```python
from build123d import *

# Parameters (mm, degrees)
F0_R          = 3
F0_R_2        = 2.5
F1_DEPTH      = 246.7
F2_R          = 2
F3_R          = 7
F6_DEPTH      = 30
F6_DEPTH_BACK = 30


# Not quite as in the source:
# - a feature names something its author has since deleted; it is built from what else it names


with BuildPart() as f1:
    # F0 (on Top) → F1 (new body)
    with BuildSketch(Plane.XY):
        with BuildLine():
            Line((18.15, -30), (30, -30))
            Line((30, -30), (30, -18.15))
            Line((30, -18.15), (27.5, -18.15))
            Line((27.5, -18.15), (27.5, -20.15))
            Line((27.5, -20.15), (21.5477069044, -20.15))
            ThreePointArc((21.5477069044, -20.15), (19.5, -15), (21.5477069044, -9.85))
            Line((21.5477069044, -9.85), (27.5, -9.85))
            Line((27.5, -9.85), (27.5, -11.85))
            Line((27.5, -11.85), (30, -11.85))
            Line((30, -11.85), (30, 11.85))
            Line((30, 11.85), (27.5, 11.85))
            Line((27.5, 11.85), (27.5, 9.85))
            Line((27.5, 9.85), (21.5477069044, 9.85))
            ThreePointArc((21.5477069044, 9.85), (19.5, 15), (21.5477069044, 20.15))
            Line((21.5477069044, 20.15), (27.5, 20.15))
            Line((27.5, 20.15), (27.5, 18.15))
            Line((27.5, 18.15), (30, 18.15))
            Line((30, 18.15), (30, 30))
            Line((30, 30), (18.15, 30))
            Line((18.15, 30), (18.15, 27.5))
            Line((18.15, 27.5), (20.15, 27.5))
            Line((20.15, 27.5), (20.15, 21.5477069044))
            ThreePointArc((20.15, 21.5477069044), (15, 19.5), (9.85, 21.5477069044))
            Line((9.85, 21.5477069044), (9.85, 27.5))
            Line((9.85, 27.5), (11.85, 27.5))
            Line((11.85, 27.5), (11.85, 30))
            Line((11.85, 30), (-11.85, 30))
            Line((-11.85, 30), (-11.85, 27.5))
            Line((-11.85, 27.5), (-9.85, 27.5))
            Line((-9.85, 27.5), (-9.85, 21.5477069044))
            ThreePointArc((-9.85, 21.5477069044), (-15, 19.5), (-20.15, 21.5477069044))
            Line((-20.15, 21.5477069044), (-20.15, 27.5))
            Line((-20.15, 27.5), (-18.15, 27.5))
            Line((-18.15, 27.5), (-18.15, 30))
            Line((-18.15, 30), (-30, 30))
            Line((-30, 30), (-30, 18.15))
            Line((-30, 18.15), (-27.5, 18.15))
            Line((-27.5, 18.15), (-27.5, 20.15))
            Line((-27.5, 20.15), (-21.5477069044, 20.15))
            ThreePointArc((-21.5477069044, 20.15), (-19.5, 15), (-21.5477069044, 9.85))
            Line((-21.5477069044, 9.85), (-27.5, 9.85))
            Line((-27.5, 9.85), (-27.5, 11.85))
            Line((-27.5, 11.85), (-30, 11.85))
            Line((-30, 11.85), (-30, -11.85))
            Line((-30, -11.85), (-27.5, -11.85))
            Line((-27.5, -11.85), (-27.5, -9.85))
            Line((-27.5, -9.85), (-21.5477069044, -9.85))
            ThreePointArc((-21.5477069044, -9.85), (-19.5, -15), (-21.5477069044, -20.15))
            Line((-21.5477069044, -20.15), (-27.5, -20.15))
            Line((-27.5, -20.15), (-27.5, -18.15))
            Line((-27.5, -18.15), (-30, -18.15))
            Line((-30, -18.15), (-30, -30))
            Line((-30, -30), (-18.15, -30))
            Line((-18.15, -30), (-18.15, -27.5))
            Line((-18.15, -27.5), (-20.15, -27.5))
            Line((-20.15, -27.5), (-20.15, -21.5477069044))
            ThreePointArc((-20.15, -21.5477069044), (-15, -19.5), (-9.85, -21.5477069044))
            Line((-9.85, -21.5477069044), (-9.85, -27.5))
            Line((-9.85, -27.5), (-11.85, -27.5))
            Line((-11.85, -27.5), (-11.85, -30))
            Line((-11.85, -30), (11.85, -30))
            Line((11.85, -30), (11.85, -27.5))
            Line((11.85, -27.5), (9.85, -27.5))
            Line((9.85, -27.5), (9.85, -21.5477069044))
            ThreePointArc((9.85, -21.5477069044), (15, -19.5), (20.15, -21.5477069044))
            Line((20.15, -21.5477069044), (20.15, -27.5))
            Line((20.15, -27.5), (18.15, -27.5))
            Line((18.15, -27.5), (18.15, -30))
        make_face()
        with Locations((-25, -25)):
            Circle(F0_R, mode=Mode.SUBTRACT)
        with Locations((-15, -15)):
            Circle(F0_R_2, mode=Mode.SUBTRACT)
        with Locations((25, -25)):
            Circle(F0_R, mode=Mode.SUBTRACT)
        with Locations((15, -15)):
            Circle(F0_R_2, mode=Mode.SUBTRACT)
        with Locations((-25, 25)):
            Circle(F0_R, mode=Mode.SUBTRACT)
        with Locations((-15, 15)):
            Circle(F0_R_2, mode=Mode.SUBTRACT)
        Polygon((-7, 22), (-7, 27.5), (0, 27.5), (7, 27.5), (7, 22), (10, 16), (10, 10), (16, 10), (22, 7), (27.5, 7), (27.5, 0), (27.5, -7), (22, -7), (16, -10), (10, -10), (10, -16), (7, -22), (7, -27.5), (0, -27.5), (-7, -27.5), (-7, -22), (-10, -16), (-10, -10), (-16, -10), (-22, -7), (-27.5, -7), (-27.5, 0), (-27.5, 7), (-22, 7), (-16, 10), (-10, 10), (-10, 16), align=None, mode=Mode.SUBTRACT)
        with Locations((15, 15)):
            Circle(F0_R_2, mode=Mode.SUBTRACT)
        with Locations((25, 25)):
            Circle(F0_R, mode=Mode.SUBTRACT)
    extrude(amount=F1_DEPTH)

    # F2
    f2_edges = [f1.edges().sort_by_distance(p)[0] for p in [
        (-7, 27.5, 123.35),
        (7, 27.5, 123.35),
    ]]
    fillet(f2_edges, radius=F2_R)

    # F3
    f3_edges = [f1.edges().sort_by_distance(p)[0] for p in [
        (-10, 16, 123.35),
        (10, 16, 123.35),
    ]]
    fillet(f3_edges, radius=F3_R)

    # F5 (on Front) → F6 (cut, two sides)
    with BuildSketch(Plane.XZ) as f6_sk:
        Polygon((-21.4844248466, -51.4844248466), (30, 0), (-30.7442165391, 60.7442165391), (-82.2286413857, 9.2597916926), align=None)
        Polygon((69.921577374, 205.311127478), (91.4664718921, 257.3251040235), (-8.4551054819, 298.7139765456), (-30, 246.7), align=None)
    extrude(amount=F6_DEPTH, mode=Mode.SUBTRACT)
    extrude(f6_sk.sketch, amount=-F6_DEPTH_BACK, mode=Mode.SUBTRACT)


solid = f1.part
```
Check sheet for the modelled part. Datum: model origin and axes. Units: mm. Give positions to 0.01 mm unless a question says otherwise; leave off trailing zeros. Order: outer loops, then holes, each group sorted by start corner. A loop starts at its lowest first (then second) coordinate and runs counter-clockwise, first axis right, second up. Notation, with made-up numbers: (43, -40) -> (87, -40) arc R24 ccw to (87, -13) -> close; hole circle Ø4 at (78, 48). An arc over 180 degrees is marked (long way). Return JSON: item names as keys, results as strings.
1. Mould release check, pull along X, two halves, no side actions. Record for faces 1 (the flat face through (-30, -24, 152)), 2 (the flat face through (0, -30, 127)), 3 (the flat face through (-19, 8.5, 143.3)), 4 (the flat face through (30, 24, 109)): +X half, -X half, draft (parallel to the pull), parting line (faces both ways), or undercut.
From the geometry:
{"face 1": "-X half", "face 2": "draft", "face 3": "undercut", "face 4": "+X half"}
2. Material ranges on probe 1 along X at (y, z) = (-15, 199); probe 2 along Y at (x, z) = (-25, 200.5); probe 3 along X at (y, z) = (4, 209.5), recorded low to high. Write a range as [from, to].
From the geometry:
{"probe 1": "[-19.5, -17.5], [-12.5, -10], [10, 12.5], [17.5, 19.5]", "probe 2": "[-30, -28], [-22, -20.15], [-9.85, -7], [7, 9.85], [20.15, 22], [28, 30]", "probe 3": "[-30, -27.5], [27.5, 30]"}
3. Cross-section at C-C, the plane z = 91. Count the separate pieces of the cut face and the enclosed holes in it, plus the area to 3 significant figures.
From the geometry:
{"separate pieces": "1", "enclosed holes": "9", "area": "1,080 mm^2"}
4. Cross-section at B-B, the plane y = -25. Record the cut outline in (x, z).
From the geometry:
{"outline": "(-30, 60) -> (-28, 58) -> (-28, 245.87) -> (-30, 246.7) -> close; (-22, 52) -> (-20.15, 50.15) -> (-20.15, 242.62) -> (-22, 243.39) -> close; (-9.85, 39.85) -> (-7, 37) -> (-7, 237.17) -> (-9.85, 238.35) -> close; (7, 23) -> (9.85, 20.15) -> (9.85, 230.19) -> (7, 231.37) -> close; (20.15, 9.85) -> (22, 8) -> (22, 225.16) -> (20.15, 225.93) -> close; (28, 2) -> (30, 0) -> (30, 221.85) -> (28, 222.68) -> close"}
5. Go/stop test with flat-tipped pins: P1, Ø1.8, axis at y = -13.5, z = 140.5, coming from the +X side; P2, Ø10, axis at x = -10, y = 7, coming from the +Z side. Record where each tip stops, or that it passes through.
From the geometry:
{"P1": "x = 19.89", "P2": "z = 240.07"}
6. Cross-section at A-A, the plane x = 0. Record the cut outline in (y, z).
From the geometry:
{"outline": "(-30, 30) -> (-27.5, 30) -> (-27.5, 234.27) -> (-30, 234.27) -> close; (27.5, 30) -> (30, 30) -> (30, 234.27) -> (27.5, 234.27) -> close"}
